from build123d import *

# Parameters (mm, degrees)
BOX001_W            = 14
BOX001_H            = 20
BOX001_DEPTH        = 10
BOX_W               = 10
BOX_H               = 20
BOX_DEPTH           = 10
BOX_PLACEMENT_ANGLE = 45


with BuildPart() as cubo001:
    # Box001 → Box001 (new body)
    with BuildSketch(Plane(origin=(-2, 0, 0), x_dir=(1, 0, 0), z_dir=(0, 0, 1))):
        with Locations((7, 10)):
            Rectangle(BOX001_W, BOX001_H)
    extrude(amount=BOX001_DEPTH)


with BuildPart() as fusion:
    # Box → Box (new body)
    with BuildSketch(Plane.XY):
        with Locations((5, 10)):
            Rectangle(BOX_W, BOX_H)
    extrude(amount=BOX_DEPTH)


with BuildPart() as fusion_1:
    # Box placement: moved
    add(fusion.part.moved(Location((-2.071068, 0, 10))).rotate(Axis((-2.071068, 0, 10), (0, 1, 0)), BOX_PLACEMENT_ANGLE))

    # Fusion: union Cubo001
    add(cubo001.part)


solid = fusion_1.part
CAD build for the part. Positions are in the model's coordinates, mm. A direction names the side the tool comes from. Coordinates: 2 decimals unless noted, no trailing zeros. Write each loop counter-clockwise with the first axis right and the second up, starting at its lowest first coordinate (ties: lowest second). Pieces come first, ordered by that corner, then holes. Notation, with made-up numbers: M -28.75,74.25 L 3.25,74.25 A30 cw 3.25,101.25 Z; hole C 4.25,81.5 d4. An arc over 180 degrees is marked long. Answer as a JSON object with one key per item and string values. Group by question number.
1) Pin check, flat tips, straight feed: pin 1 Ø6 at (y, z) = (16.5, 12.5) entering from +X; pin 2 Ø8 at (y, z) = (6.5, 3) entering from +X; pin 3 Ø3 at (y, z) = (14.5, 3) entering from -X. Stop position of each tip, or through.
2) Mould opens along Z. For faces 3 (the face through (12, 10, 5)), 4 (the face through (5, 10, 0)), 5 (the face through (1.415, 9.86, 13.486)) say: +Z half, -Z half, draft (parallel to the pull), parting line (faces both ways), or undercut.
3) Saw through at C-C (z = 13.5). Write the cut outline in (x, y), plus the area to 3 significant figures.
4) Wall check: line 1 (X direction, y = 7.75, z = 9); line 2 (Z direction, x = 8, y = 7); line 3 (Z direction, x = 3, y = 15.5). Give the ranges that are in metal, low to high. Write a range as from..to.
5) Tool access for faces 1 (the face through (-2, 10, 5)), 2 (the face through (5, 0, 7)): list every direction of +Z, -Z, +X, -X, +Y, -Y with a clear straight run to the whole face (end or side of a thin tool).
6) Saw through at B-B (x = -1). Write the cut outline in (y, z).
7) Saw through at A-A (y = 11.5). Write the cut outline in (x, z), plus the area to 3 significant figures.
Values follow:
{
 "1": {"pin 1": "stops at x = 12.07", "pin 2": "stops at x = 12", "pin 3": "stops at x = -2"},
 "2": {"face 3": "draft", "face 4": "-Z half", "face 5": "+Z half"},
 "3": {"outline": "M 1.43,0 L 8.57,0 L 8.57,20 L 1.43,20 Z", "area": "143 mm2"},
 "4": {"line 1": "x = -2..12", "line 2": "z = 0..14.07", "line 3": "z = 0..15.07"},
 "5": {"face 1": "-Z, -X, +Y, -Y", "face 2": "+Z, -Z, +X, -X, -Y"},
 "6": {"outline": "M 0,0 L 20,0 L 20,11.07 L 0,11.07 Z"},
 "7": {"outline": "M -2.07,10 L -2,9.93 L -2,0 L 12,0 L 12,9.93 L 12.07,10 L 5,17.07 Z", "area": "190 mm2"}
}
